Job drawing, mm, ordinate dimensions from the low corner. One solid piece. A direction names the side the tool comes from. Round coordinates to 2 decimals unless told otherwise and drop trailing zeros. Loops run counter-clockwise (first coordinate to the right, second up) from the corner with the lowest first, then second, coordinate; pieces in that order, holes last.
1) Mould opens along Y. For the marked faces 4, 5 and 6 say: +Y half, -Y half, draft (parallel to the pull), parting line (faces both ways), or undercut.
2) Band-saw the part on A-A, the plane z = 27. Write the cut outline in (x, y), then the cut area to 3 significant figures.
3) Drop flat-ended pins along their axis: P1, Ø1.5, axis at y = 53.5, z = 15, coming from the -X side; P2, Ø9, axis at x = 11, z = 9, coming from the -Y side; P3, Ø8, axis at y = 42.5, z = 16, coming from the +X side; P4, Ø1, axis at x = 12, y = 52.5, coming from the +Z side. Give the stop position or say it passes through.
4) Band-saw the part on C-C, the plane y = 24. Write the cut outline in (x, z), then the cut area to 3 significant figures.
5) Band-saw the part on D-D, the plane z = 14.75. Write the cut outline in (x, y), then the cut area to 3 significant figures.
6) Probe line 1 (Y direction, x = 26, z = 24.75); line 2 (Y direction, x = 23.5, z = 14); line 3 (X direction, y = 18, z = 14.5). List the from-to ranges inside material, lowest first.
7) Band-saw the part on B-B, the plane x = 15. Write the cut outline in (y, z), then the cut area to 3 significant figures.
8) 3-axis set-ups, long thin cutter, end or side, ignore diameter. For the marked faces 1, 2 and 3: which of +Z, -Z, +X, -X, +Y, -Y reach the whole face in a straight line?
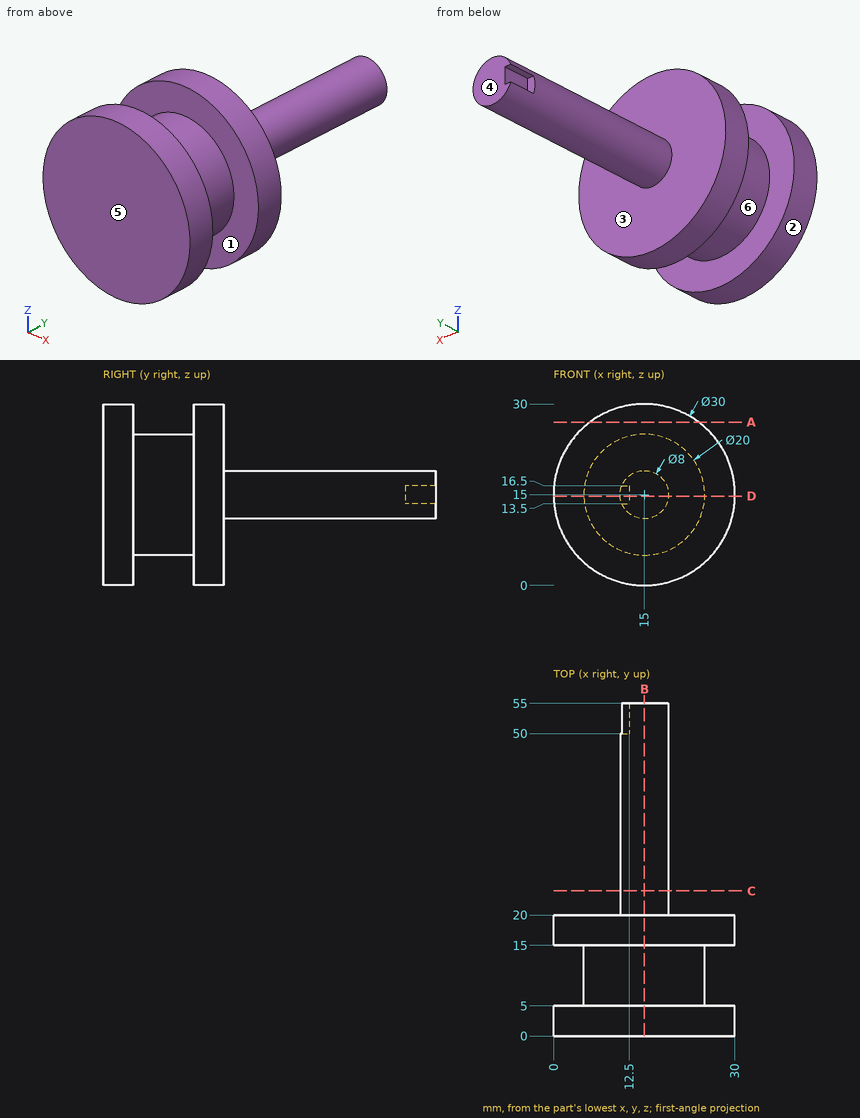
Reported:
1. face 4: +Y half
1. face 5: -Y half
1. face 6: undercut
2. outline: (6, 0) - (24, 0) - (24, 5) - (6, 5) - close; (6, 15) - (24, 15) - (24, 20) - (6, 20) - close
2. area: 180 mm2
3. P1: stops at x = 12.5
3. P2: stops at y = 0
3. P3: stops at x = 19
3. P4: stops at z = 18.12
4. outline: circle Ø8 at (15, 15)
4. area: 50.3 mm2
5. outline: (0, 0) - (30, 0) - (30, 5) - (25, 5) - (25, 15) - (30, 15) - (30, 20) - (18.99, 20) - (18.99, 55) - (12.5, 55) - (12.5, 50) - (11.01, 50) - (11.01, 20) - (0, 20) - (0, 15) - (5, 15) - (5, 5) - (0, 5) - close
5. area: 772 mm2
6. line 1: y = 0 to 5, 15 to 20
6. line 2: y = 0 to 20
6. line 3: x = 0.01 to 29.99
7. outline: (0, 0) - (5, 0) - (5, 5) - (15, 5) - (15, 0) - (20, 0) - (20, 11) - (55, 11) - (55, 19) - (20, 19) - (20, 30) - (15, 30) - (15, 25) - (5, 25) - (5, 30) - (0, 30) - close
7. area: 780 mm2
8. face 1: none
8. face 2: +Y, -Y
8. face 3: +Y
